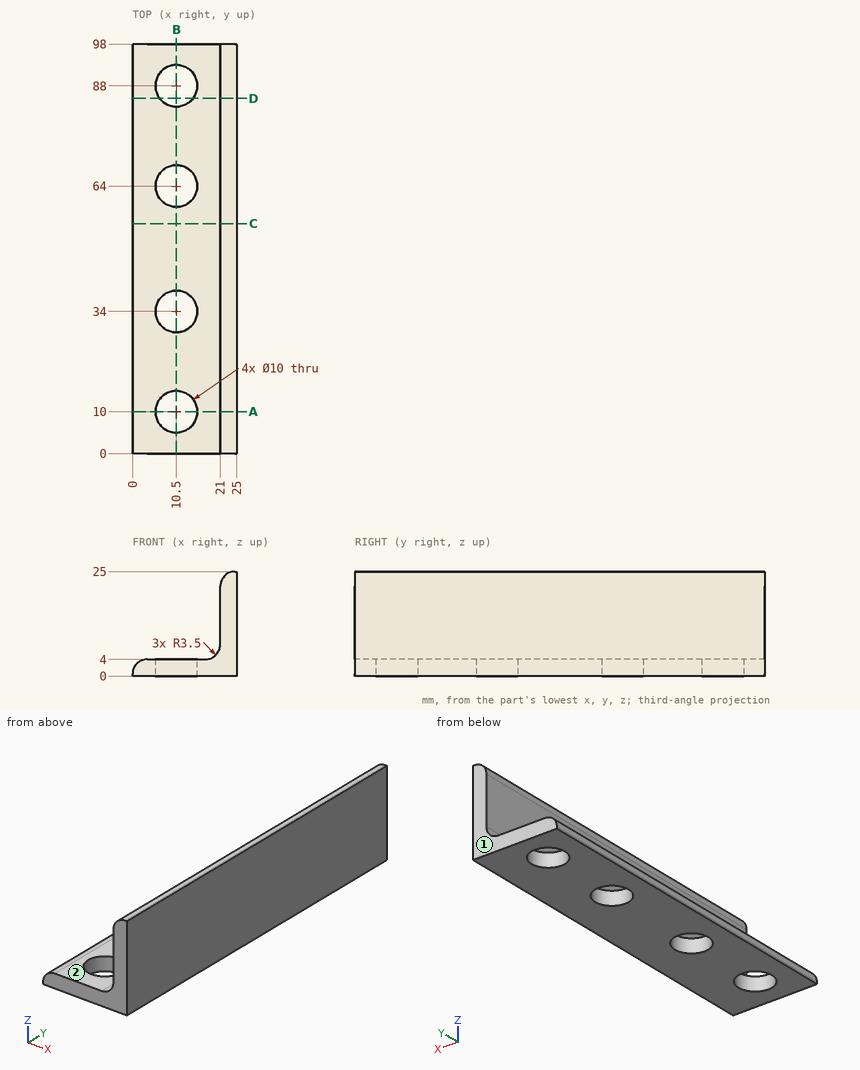
Study the drawing (mm; zero at the part's minimum x, y, z) and answer. A direction names the side the tool comes from. Give positions to 0.01 mm unless a question says otherwise; leave off trailing zeros. Loops run counter-clockwise (first coordinate to the right, second up) from the corner with the lowest first, then second, coordinate; pieces in that order, holes last. Notation, with made-up numbers: M 15.5,53 L 63.5,53 A17 cw 63.5,58 Z; hole C 31,61.5 d7. An arc over 180 degrees is marked long. Answer as CSV lines item,"result".
Item 1: The part is cut by section A-A (y = 10). Give the vertices of the cut face in (x, z), and give its area (3 significant figures).
Values follow:
outline,"M 0,0 L 5.5,0 L 5.5,4 L 3.5,4 A3.5 ccw 0,0.5 Z; M 15.5,0 L 25,0 L 25,25 L 24.5,25 A3.5 ccw 21,21.5 L 21,7.5 A3.5 cw 17.5,4 L 15.5,4 Z"
area,"141 mm^2"
Item 2: The part is cut by section D-D (y = 85). Give the vertices of the cut face in (x, z), and give its area (3 significant figures).
Values follow:
outline,"M 0,0 L 6.5,0 L 6.5,4 L 3.5,4 A3.5 ccw 0,0.5 Z; M 14.5,0 L 25,0 L 25,25 L 24.5,25 A3.5 ccw 21,21.5 L 21,7.5 A3.5 cw 17.5,4 L 14.5,4 Z"
area,"149 mm^2"
Item 3: Which of the six approach directions +Z, -Z, +X, -X, +Y, -Y give full straight-line access (tool end or side, diameter ignored) to the marked faces 1 and 2?
Values follow:
face 1,"+Z, -Z, +X, -X, +Y"
face 2,"+Z, -X, +Y, -Y"
Item 4: Given pin 1 Ø1 at (x, y) = (7, 35) entering from -Z; pin 2 Ø10 at (x, y) = (10.5, 53.5) entering from +Z; pin 3 Ø11 at (y, z) = (33.5, 12) entering from -X, each flat-ended and moving along its own axis, determine where each tip first touches the part or whether it passes through.
Values follow:
pin 1,"passes through"
pin 2,"stops at z = 4"
pin 3,"stops at x = 20.85"
Item 5: The part is cut by section C-C (y = 55). Give the vertices of the cut face in (x, z), and give its area (3 significant figures).
Values follow:
outline,"M 0,0 L 25,0 L 25,25 L 24.5,25 A3.5 ccw 21,21.5 L 21,7.5 A3.5 cw 17.5,4 L 3.5,4 A3.5 ccw 0,0.5 Z"
area,"181 mm^2"
Item 6: The part is cut by section B-B (x = 10.5). Give the vertices of the cut face in (y, z), and give its area (3 significant figures).
Values follow:
outline,"M 0,0 L 5,0 L 5,4 L 0,4 Z; M 15,0 L 29,0 L 29,4 L 15,4 Z; M 39,0 L 59,0 L 59,4 L 39,4 Z; M 69,0 L 83,0 L 83,4 L 69,4 Z; M 93,0 L 98,0 L 98,4 L 93,4 Z"
area,"232 mm^2"
Item 7: Straight lines are drawn through the part: line 1 along Y through (x, z) = (10.5, 1.75); line 2 along Z through (x, y) = (4.75, 17); line 3 along X through (y, z) = (53.5, 14.75). For each, find the intervals that lie inside material, in ascending order. Write a range as [from, to].
Values follow:
line 1,"y = [0, 5], [15, 29], [39, 59], [69, 83], [93, 98]"
line 2,"z = [0, 4]"
line 3,"x = [21, 25]"
